Could you check a few things on this model? Use its own coordinates, in mm. Face numbers are marked on the shaded views. A direction names the side the tool comes from. Coordinates: 2 decimals unless noted, no trailing zeros. Order: outer loops, then holes, each group sorted by start corner. A loop starts at its lowest first (then second) coordinate and runs counter-clockwise, first axis right, second up. Notation, with made-up numbers: (35.5, -20) - (45.5, -20) arc R28 ccw to (45.5, 3) - close; hole circle Ø1 at (-15, -10.5). An arc over 180 degrees is marked (long way). One line per item, written item: value.
from build123d import *

# Parameters (mm, degrees)
SKETCH_1_W      = 19.5
SKETCH_1_H      = 5
SKETCH_1_W_2    = 17.5
SKETCH_1_H_2    = 3
EXTRUDE_1_DEPTH = 5
FILLET_1_R      = 2.2
FILLET_2_R      = 1
FILLET_3_R      = 0.2


with BuildPart() as part:
    # Эскиз1 → Бобышка-Вытянуть1 (new body)
    with BuildSketch(Plane.XY):
        Rectangle(SKETCH_1_W, SKETCH_1_H)
        Rectangle(SKETCH_1_W_2, SKETCH_1_H_2, mode=Mode.SUBTRACT)
    extrude(amount=EXTRUDE_1_DEPTH)

    # Скругление1
    fillet_1_edges = [part.edges().sort_by_distance(p)[0] for p in [
        (-9.75, 2.5, 2.5),
        (9.75, 2.5, 2.5),
        (9.75, -2.5, 2.5),
        (-9.75, -2.5, 2.5),
    ]]
    fillet(fillet_1_edges, radius=FILLET_1_R)

    # Скругление2
    fillet_2_edges = [part.edges().sort_by_distance(p)[0] for p in [
        (8.75, -1.5, 2.5),
        (-8.75, -1.5, 2.5),
    ]]
    fillet(fillet_2_edges, radius=FILLET_2_R)

    # Скругление3
    fillet_3_edges = [part.edges().sort_by_distance(p)[0] for p in [
        (-8.75, 0.5, 0),
        (-8.75, 0.5, 5),
        (0, 2.5, 0),
        (0, 2.5, 5),
        (-9.75, 0, 0),
        (9.75, 0, 0),
        (0, -2.5, 0),
        (9.105634919, -1.855634919, 0),
        (-9.105634919, -1.855634919, 0),
        (-9.105634919, 1.855634919, 0),
        (9.105634919, 1.855634919, 0),
        (9.75, 0, 5),
        (-9.75, 0, 5),
        (0, -2.5, 5),
        (9.105634919, -1.855634919, 5),
        (-9.105634919, -1.855634919, 5),
        (-9.105634919, 1.855634919, 5),
        (9.105634919, 1.855634919, 5),
        (0, -1.5, 0),
        (0, -1.5, 5),
        (8.75, 0.5, 0),
        (8.75, 0.5, 5),
        (-8.457106781, -1.207106781, 0),
        (-8.457106781, -1.207106781, 5),
        (8.457106781, -1.207106781, 0),
        (8.457106781, -1.207106781, 5),
    ]]
    fillet(fillet_3_edges, radius=FILLET_3_R)


solid = part.part
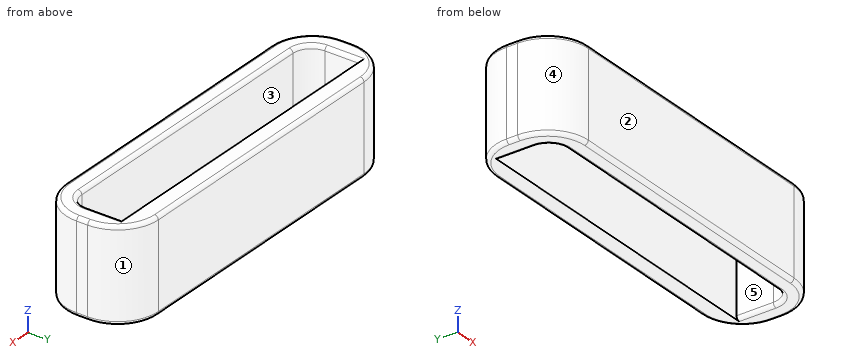
Item 1: If I drill on probe 1 along Y at (x, z) = (-4.25, 1.6); probe 2 along X at (y, z) = (0.2, 3.55); probe 3 along X at (y, z) = (2, 2.55), over which ranges is the centre line in solid material (lowest first)?
Conclusion:
probe 1: -2.5 to -1.5, 1.5 to 2.5
probe 2: -9.75 to -8.75, 8.75 to 9.75
probe 3: -8.95 to 8.95
Item 2: I want a section at A-A on x = -3.25. Please give me the cut outline in (y, z), then the cut area to 3 significant figures.
Conclusion:
outline: (-2.5, 0.2) arc R0.2 ccw to (-2.3, 0) - (-1.7, 0) arc R0.2 ccw to (-1.5, 0.2) - (-1.5, 4.8) arc R0.2 ccw to (-1.7, 5) - (-2.3, 5) arc R0.2 ccw to (-2.5, 4.8) - close; (1.5, 0) - (2.3, 0) arc R0.2 ccw to (2.5, 0.2) - (2.5, 4.8) arc R0.2 ccw to (2.3, 5) - (1.5, 5) - close
area: 9.95 mm²
Item 3: Thinking about a two-plate mould opening in X: for the marked faces 1, 2 and 3, which applies, pulls with the +X half, pulls with the -X half, needs draft (parallel to the pull), parting line crosses it, or undercut?
Conclusion:
face 1: pulls with the +X half
face 2: needs draft
face 3: undercut
Item 4: For the marked faces 4 and 5, which set-ups out of +Z, -Z, +X, -X, +Y, -Y let a thin tool reach every point of the face, with its end or its side?
Conclusion:
face 4: +Z, -Z, -X, -Y
face 5: +Z, -Z
Item 5: I want a section at B-B on z = 3.65. Please give me the cut outline in (x, y).
Conclusion:
outline: (-9.75, -0.3) arc R2.2 ccw to (-7.55, -2.5) - (7.55, -2.5) arc R2.2 ccw to (9.75, -0.3) - (9.75, 0.3) arc R2.2 ccw to (7.55, 2.5) - (-7.55, 2.5) arc R2.2 ccw to (-9.75, 0.3) - close; hole (-8.75, -0.5) arc R1 ccw to (-7.75, -1.5) - (7.75, -1.5) arc R1 ccw to (8.75, -0.5) - (8.75, 1.5) - (-8.75, 1.5) - close
